Build history of the part. All positions in model axes, mm. Face numbers are marked on the shaded views. A direction names the side the tool comes from. Give positions to 0.01 mm unless a question says otherwise; leave off trailing zeros. Write each loop counter-clockwise with the first axis right and the second up, starting at its lowest first coordinate (ties: lowest second). Pieces come first, ordered by that corner, then holes. Notation, with made-up numbers: (5.5, 31) -> (50.5, 31) arc R20 cw to (50.5, 70) -> close; hole circle Ø2 at (77.5, -16). An arc over 180 degrees is marked (long way). Put each result on its own line as item: value. Start each with the question number.
Item 1: Slice it at D-D, the plane y = 20. List the corners of the cut face in (x, z), plus the area to 3 significant figures.
Item 2: Two-plate mould, pull along Y, no slides. Class the marked faces 4, 5, 6 and 7: pulls with the +Y half, pulls with the -Y half, needs draft (parallel to the pull), parting line crosses it, or undercut.
Item 3: Slice it at C-C, the plane x = 20.5. List the corners of the cut face in (y, z), plus the area to 3 significant figures.
Item 4: Slice it at A-A, the plane y = 13. List the corners of the cut face in (x, z).
Item 5: Tool access for the marked faces 1, 2 and 3: list every direction of +Z, -Z, +X, -X, +Y, -Y with a clear straight run to the whole face (end or side of a thin tool).
Item 6: Slice it at B-B, the plane x = 10.5. List the corners of the cut face in (y, z), plus the area to 3 significant figures.
Item 7: Flat gauge pins, fed straight in: pin 1 Ø3 at (y, z) = (8, -6.5) entering from -X; pin 2 Ø0.6 at (x, z) = (17.5, -1) entering from +Y; pin 3 Ø2 at (y, z) = (18, -1.5) entering from -X; pin 4 Ø8 at (x, y) = (27, 12.5) entering from -Z. Where does each tip first touch, or does it go through?
Item 8: Drill centre lines: line 1 along Z through (x, y) = (6.75, 11.25); line 2 along Y through (x, z) = (12.25, -4.75); line 3 along Y through (x, z) = (17.5, -7). Where is each one in solid material? Low to high.
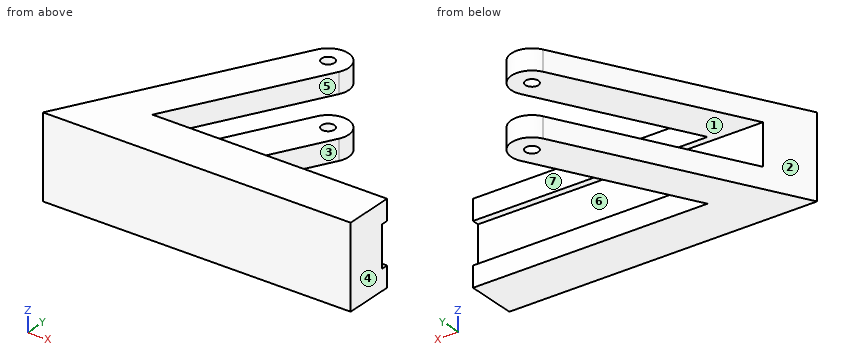
```python
from build123d import *

# Parameters (mm, degrees)
EXTRUDE_1_DEPTH     = 8
SKETCH_2_W          = 4
SKETCH_2_H          = 18.866305448
CUT_EXTRUDE_1_DEPTH = 88
SKETCH_3_R          = 0.625
CUT_EXTRUDE_2_DEPTH = 88


with BuildPart() as part:
    # 草圖1 → 填料-伸長1 (new body)
    with BuildSketch(Plane.XY):
        with BuildLine():
            Line((0, 0), (11.292732867, 20.94901356))
            ThreePointArc((11.292732867, 20.94901356), (14.002250122, 21.760503696), (14.813740258, 19.05098644))
            Line((14.813740258, 19.05098644), (7.13506975, 4.806376698))
            Line((7.13506975, 4.806376698), (30, 4.806376698))
            Line((30, 4.806376698), (30, 0))
            Line((30, 0), (0, 0))
        make_face()
    extrude(amount=-EXTRUDE_1_DEPTH)

    # 草圖2 → 除料-伸長1 (cut)
    with BuildSketch(Plane(origin=(30, 0, 0), x_dir=(0, 0, -1), z_dir=(1, 0, 0))):
        with Locations((4, 13.566847276)):
            Rectangle(SKETCH_2_W, SKETCH_2_H)
    extrude(amount=-CUT_EXTRUDE_1_DEPTH, mode=Mode.SUBTRACT)

    # 草圖3 → 除料-伸長2 (cut)
    with BuildSketch(Plane.XY):
        with Locations(Location((13.053236562, 20, 0), (0, 0, 180))):
            Circle(SKETCH_3_R)
    extrude(amount=-CUT_EXTRUDE_2_DEPTH, mode=Mode.SUBTRACT)


solid = part.part
```
Values follow:
1. outline: (10.78, -8) -> (12.43, -8) -> (12.43, -6) -> (10.78, -6) -> close; (10.78, -2) -> (12.43, -2) -> (12.43, 0) -> (10.78, 0) -> close; (13.68, -8) -> (15.05, -8) -> (15.05, -6) -> (13.68, -6) -> close; (13.68, -2) -> (15.05, -2) -> (15.05, 0) -> (13.68, 0) -> close
1. area: 12.1 mm2
2. face 4: needs draft
2. face 5: undercut
2. face 6: pulls with the +Y half
2. face 7: undercut
3. outline: (0, -8) -> (4.81, -8) -> (4.81, -6) -> (4.13, -6) -> (4.13, -2) -> (4.81, -2) -> (4.81, 0) -> (0, 0) -> close
3. area: 35.8 mm2
4. outline: (7.01, -8) -> (11.55, -8) -> (11.55, -6) -> (7.01, -6) -> close; (7.01, -2) -> (11.55, -2) -> (11.55, 0) -> (7.01, 0) -> close
5. face 1: +X, -X, +Y
5. face 2: +Z, -Z, -X, +Y
5. face 3: +Z, -Z, +X
6. outline: (0, -8) -> (4.81, -8) -> (4.81, -6) -> (4.13, -6) -> (4.13, -2) -> (4.81, -2) -> (4.81, 0) -> (0, 0) -> close; (11.05, -8) -> (19.48, -8) -> (19.48, -6) -> (11.05, -6) -> close; (11.05, -2) -> (19.48, -2) -> (19.48, 0) -> (11.05, 0) -> close
6. area: 69.5 mm2
7. pin 1: x = 3.5
7. pin 2: y = 4.81
7. pin 3: x = 9.16
7. pin 4: through
8. line 1: -8 to -6, -2 to 0
8. line 2: 0 to 4.13
8. line 3: 0 to 4.81
